from build123d import *

# Parameters (mm, degrees)
SKETCH_W        = 90.5
SKETCH_H        = 62.5
PAD_DEPTH       = 22.6
SKETCH001_W     = 85.5
SKETCH001_H     = 56.5
POCKET_DEPTH    = 20.6
SKETCH002_W     = 15
SKETCH002_H     = 16
SKETCH002_W_2   = 16.3
POCKET001_DEPTH = 5
SKETCH003_R     = 3
PAD001_DEPTH    = 3
SKETCH004_R     = 1.6
POCKET002_DEPTH = 5
SKETCH005_R     = 2.65
POCKET003_DEPTH = 2.5
CHAMFER_SIZE    = 0.7
SKETCH006_W     = 61
SKETCH006_H     = 3
POCKET004_DEPTH = 7.6
SKETCH007_W     = 21.5
SKETCH007_H     = 1.5
POCKET005_DEPTH = 3
SKETCH008_W     = 3
SKETCH008_H     = 1.5
POCKET006_DEPTH = 3
SKETCH009_W     = 1.5
SKETCH009_H     = 58
POCKET007_DEPTH = 3
SKETCH010_W     = 87
SKETCH010_H     = 1.5
POCKET008_DEPTH = 3
CHAMFER001_SIZE = 1
FILLET_R        = 3
SKETCH011_W     = 9
SKETCH011_H     = 8
SKETCH011_W_2   = 16
SKETCH011_W_3   = 7
POCKET009_DEPTH = 5
SKETCH012_W     = 52.4
SKETCH012_H     = 16
POCKET010_DEPTH = 5
SKETCH013_W     = 13.003716
SKETCH013_H     = 12
POCKET011_DEPTH = 8


with BuildPart() as part:
    # Sketch → Pad (new body)
    with BuildSketch(Plane.XY):
        Rectangle(SKETCH_W, SKETCH_H)
    extrude(amount=PAD_DEPTH)

    # Sketch001 (on Face6 of Pad) → Pocket (cut)
    with BuildSketch(Plane.XY.offset(22.6)):
        with Locations((-0.5, 0)):
            Rectangle(SKETCH001_W, SKETCH001_H)
    extrude(amount=-POCKET_DEPTH, mode=Mode.SUBTRACT)

    # Sketch002 (on Face2 of Pocket) → Pocket001 (cut)
    with BuildSketch(Plane(origin=(-45.25, 0, 0), x_dir=(0, -1, 0), z_dir=(-1, 0, 0))):
        with Locations((19, 14.6)):
            Rectangle(SKETCH002_W, SKETCH002_H)
        with Locations((1, 14.6)):
            Rectangle(SKETCH002_W, SKETCH002_H)
        with Locations((-17.75, 14.6)):
            Rectangle(SKETCH002_W_2, SKETCH002_H)
    extrude(amount=-POCKET001_DEPTH, mode=Mode.SUBTRACT)

    # Sketch003 (on Face22 of Pocket001) → Pad001 (join)
    with BuildSketch(Plane.XY.offset(2)):
        with Locations((-19.5, 24.5)):
            Circle(SKETCH003_R)
        with Locations((38.5, 24.5)):
            Circle(SKETCH003_R)
        with Locations((-19.5, -24.5)):
            Circle(SKETCH003_R)
        with Locations((38.5, -24.5)):
            Circle(SKETCH003_R)
    extrude(amount=PAD001_DEPTH)

    # Sketch004 (on Face30 of Pad001) → Pocket002 (cut)
    with BuildSketch(Plane.XY.offset(5)):
        with Locations((-19.5, 24.5)):
            Circle(SKETCH004_R)
        with Locations((38.5, 24.5)):
            Circle(SKETCH004_R)
        with Locations((-19.5, -24.5)):
            Circle(SKETCH004_R)
        with Locations((38.5, -24.5)):
            Circle(SKETCH004_R)
    extrude(amount=-POCKET002_DEPTH, mode=Mode.SUBTRACT)

    # Sketch005 (on Face4 of Pocket002) → Pocket003 (cut)
    with BuildSketch(Plane(origin=(0, 0, 0), x_dir=(1, 0, 0), z_dir=(0, 0, -1))):
        with Locations((38.5, 24.5)):
            Circle(SKETCH005_R)
        with Locations((-19.5, 24.5)):
            Circle(SKETCH005_R)
        with Locations((-19.5, -24.5)):
            Circle(SKETCH005_R)
        with Locations((38.5, -24.5)):
            Circle(SKETCH005_R)
    extrude(amount=-POCKET003_DEPTH, mode=Mode.SUBTRACT)

    # Chamfer
    chamfer_edges = [part.edges().sort_by_distance(p)[0] for p in [
        (-22.5, -24.5, 2),
        (35.5, -24.5, 2),
        (-22.5, 24.5, 2),
        (35.5, 24.5, 2),
    ]]
    chamfer(chamfer_edges, length=CHAMFER_SIZE)

    # Sketch006 (on Face11 of Chamfer) → Pocket004 (cut)
    with BuildSketch(Plane.XY.offset(22.6)):
        with Locations((8.75, 29.75)):
            Rectangle(SKETCH006_W, SKETCH006_H)
    extrude(amount=-POCKET004_DEPTH, mode=Mode.SUBTRACT)

    # Sketch007 (on Face11 of Pocket004) → Pocket005 (cut)
    with BuildSketch(Plane.XY.offset(22.6)):
        with Locations((-32.5, 29)):
            Rectangle(SKETCH007_W, SKETCH007_H)
    extrude(amount=-POCKET005_DEPTH, mode=Mode.SUBTRACT)

    # Sketch008 (on Face15 of Pocket005) → Pocket006 (cut)
    with BuildSketch(Plane.XY.offset(22.6)):
        with Locations((40.75, 29)):
            Rectangle(SKETCH008_W, SKETCH008_H)
    extrude(amount=-POCKET006_DEPTH, mode=Mode.SUBTRACT)

    # Sketch009 (on Face16 of Pocket006) → Pocket007 (cut)
    with BuildSketch(Plane.XY.offset(22.6)):
        with Locations((43, 0.75)):
            Rectangle(SKETCH009_W, SKETCH009_H)
    extrude(amount=-POCKET007_DEPTH, mode=Mode.SUBTRACT)

    # Sketch010 (on Face16 of Pocket007) → Pocket008 (cut)
    with BuildSketch(Plane.XY.offset(22.6)):
        with Locations((0.25, -29)):
            Rectangle(SKETCH010_W, SKETCH010_H)
    extrude(amount=-POCKET008_DEPTH, mode=Mode.SUBTRACT)

    # Chamfer001
    chamfer001_edges = [part.edges().sort_by_distance(p)[0] for p in [
        (-43.25, -11.5, 14.6),
        (-43.25, -8.5, 14.6),
        (-43.25, 6.5, 14.6),
        (-43.25, 9.6, 14.6),
        (-43.25, 25.9, 14.6),
        (-43.25, -26.5, 14.6),
    ]]
    chamfer(chamfer001_edges, length=CHAMFER001_SIZE)

    # Fillet
    fillet_edges = [part.edges().sort_by_distance(p)[0] for p in [
        (-45.25, -31.25, 11.3),
        (45.25, -31.25, 11.3),
        (-45.25, 31.25, 11.3),
        (45.25, 31.25, 11.3),
    ]]
    fillet(fillet_edges, radius=FILLET_R)

    # Sketch011 (on Face13 of Fillet) → Pocket009 (cut)
    with BuildSketch(Plane(origin=(0, 31.25, 0), x_dir=(-1, 0, 0), z_dir=(0, 1, 0))):
        with Locations((-31.65, 11)):
            Rectangle(SKETCH011_W, SKETCH011_H)
        with Locations((-10.25, 11)):
            Rectangle(SKETCH011_W_2, SKETCH011_H)
        with Locations((11.25, 11)):
            Rectangle(SKETCH011_W_3, SKETCH011_H)
    extrude(amount=-POCKET009_DEPTH, mode=Mode.SUBTRACT)

    # Sketch012 (on Face2 of Pocket009) → Pocket010 (cut)
    with BuildSketch(Plane(origin=(-45.25, 0, 0), x_dir=(0, -1, 0), z_dir=(-1, 0, 0))):
        with Locations((0.3, 14.6)):
            Rectangle(SKETCH012_W, SKETCH012_H)
    extrude(amount=-POCKET010_DEPTH, mode=Mode.SUBTRACT)

    # Sketch013 (on Face19 of Pocket010) → Pocket011 (cut)
    with BuildSketch(Plane(origin=(0, 0, 0), x_dir=(1, 0, 0), z_dir=(0, 0, -1))):
        with Locations((38.748142, 0)):
            Rectangle(SKETCH013_W, SKETCH013_H)
    extrude(amount=-POCKET011_DEPTH, mode=Mode.SUBTRACT)


solid = part.part
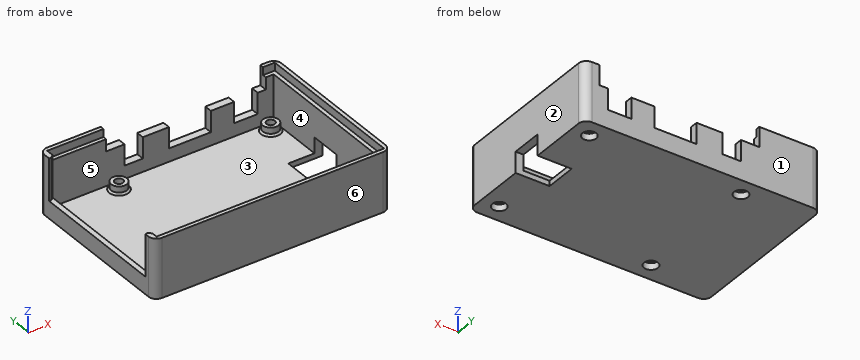
Geometry: final body of the model. Coordinates: model frame, mm. Face numbers are marked on the shaded views. A direction names the side the tool comes from. Round coordinates to 2 decimals unless told otherwise and drop trailing zeros. Order: outer loops, then holes, each group sorted by start corner. A loop starts at its lowest first (then second) coordinate and runs counter-clockwise, first axis right, second up. Notation, with made-up numbers: (-28.75, 28.25) -> (-1.75, 28.25) arc R26 ccw to (-1.75, 50.25) -> close; hole circle Ø11 at (21.25, -15.5). An arc over 180 degrees is marked (long way). Put each result on its own line as item: value. Start each with the question number.
Q1. First-contact query: pin 1 (2.5 mm diameter, centred on y = 30, z = 9.5, fed in from +X); pin 2 (1.5 mm diameter, centred on x = -22.5, y = 16.5, fed in from +Z); pin 3 (0.9 mm diameter, centred on x = 12, y = 29.5, fed in from +Z). Flat tips, straight axial feed; report the tip coordinate or a pass-through.
Q2. Section B-B on y = 2.5. Return the cut outline in (x, z), and give its area (3 significant figures).
Q3. Line query: probe 1 along Y at (x, z) = (38.5, 4.35); probe 2 along X at (y, z) = (24.5, 1.75); probe 3 along Y at (x, z) = (40, 21.5). Output: solid intervals per line, ascending.
Q4. Reachability of the marked faces 5 and 6 from +Z, -Z, +X, -X, +Y, -Y: full face, straight path, thin tool, end or side. Return the list, or none.
Q5. Section A-A on z = 12.5. Give the number of separate pieces and of enclosed holes in the cut face, and give its area (3 significant figures).
Q6. Section C-C on x = -35.5. Return the cut outline in (y, z).
Q7. Pull-direction query (X, two-part tool) for the marked faces 1, 2, 3 and 4; classes: +X half, -X half, draft (parallel to the pull), parting line (faces both ways), or undercut.
Ans:
1. pin 1: stops at x = 45.21
1. pin 2: stops at z = 2
1. pin 3: stops at z = 7
2. outline: (-45.25, 0) -> (32.25, 0) -> (32.25, 2) -> (-43.25, 2) -> (-43.25, 6.6) -> (-45.25, 6.6) -> close; (42.25, 8) -> (45.25, 8) -> (45.25, 22.6) -> (43.75, 22.6) -> (43.75, 19.6) -> (42.25, 19.6) -> close
2. area: 203 mm2
3. probe 1: y = -31.25 to -28.25, -27.5 to -26.1, -22.9 to -21.5, 21.5 to 22.9, 26.1 to 27.5, 28.25 to 31.25
3. probe 2: x = -45.25 to -22.15, -16.85 to 35.85, 41.15 to 45.25
3. probe 3: y = -31.25 to -29.75, 29.75 to 31.25
4. face 5: +Z
4. face 6: +Z, -Z, +X, -X, -Y
5. separate pieces: 4
5. enclosed holes: 0
5. area: 616 mm2
6. outline: (-31.25, 0) -> (31.25, 0) -> (31.25, 22.6) -> (29.75, 22.6) -> (29.75, 19.6) -> (28.25, 19.6) -> (28.25, 2) -> (-28.25, 2) -> (-28.25, 19.6) -> (-29.75, 19.6) -> (-29.75, 22.6) -> (-31.25, 22.6) -> close
7. face 1: draft
7. face 2: +X half
7. face 3: undercut
7. face 4: undercut
